Geometry check sheet. Reference: the model listing, model coordinates, mm. Face numbers are marked on the shaded views. Round coordinates to 2 decimals unless told otherwise and drop trailing zeros. Order: outer loops, then holes, each group sorted by start corner. A loop starts at its lowest first (then second) coordinate and runs counter-clockwise, first axis right, second up. Notation, with made-up numbers: (43, -0.5) - (75, -0.5) arc R28 ccw to (75, 21.5) - close; hole circle Ø9 at (33.25, -26). An arc over 180 degrees is marked (long way). Return JSON: item names as keys, results as strings. Group by question number.
Q1. Material ranges on line 1 along Y through (x, z) = (-5.5, 0.6); line 2 along Y through (x, z) = (-5, 1); line 3 along Z through (x, y) = (199, 3), recorded low to high.
Q2. Sectioned sample at B-B, the plane x = 130. Record the cut outline in (y, z).
Q3. Draft check along Y on the marked faces 1, 2 and 3. Enter one of: pulls with the +Y half, pulls with the -Y half, needs draft (parallel to the pull), parting line crosses it, or undercut.
Q4. Sectioned sample at A-A, the plane x = 307.5. Record the cut outline in (y, z).
Q5. Gauge pin test, flat ends, axial feed: pin 1 Ø3.5 at (x, z) = (340, 9) entering from -Y; pin 2 Ø2 at (x, z) = (-16, 7.5) entering from -Y; pin 3 Ø5 at (x, y) = (343, -4.5) entering from -Z; pin 4 Ø2.5 at (x, z) = (274, -24) entering from +Y. Record the tip position at first contact, or that the pin passes through.
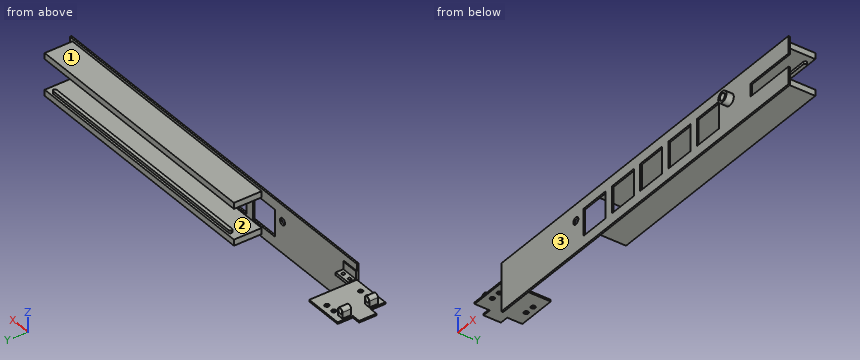
```python
from build123d import *

# Parameters (mm, degrees)
CROQUIS1_W               = 45
CROQUIS1_H               = 55
CROQUIS1_R               = 2.5
SALIENTE_EXTRUIR1_DEPTH  = 2
CROQUIS2_W               = 10
CROQUIS2_H               = 20
SALIENTE_EXTRUIR2_DEPTH  = 2
CROQUIS4_R               = 3
SALIENTE_EXTRUIR4_DEPTH  = 10
CROQUIS6_W               = 2
CROQUIS6_H               = 10
SALIENTE_EXTRUIR6_DEPTH  = 20
CROQUIS7_W               = 455
CROQUIS7_H               = 55
SALIENTE_EXTRUIR7_DEPTH  = 2
CROQUIS8_W               = 60
CROQUIS8_H               = 15
CORTAR_EXTRUIR1_DEPTH    = 2
SALIENTE_EXTRUIR8_DEPTH  = 20
CROQUIS10_R              = 1.75
CORTAR_EXTRUIR2_DEPTH    = 480.688961724
CROQUIS11_W              = 300
CROQUIS11_H              = 7
SALIENTE_EXTRUIR9_DEPTH  = 32
SALIENTE_EXTRUIR10_DEPTH = 3
CROQUIS17_R              = 4
CORTAR_EXTRUIR4_DEPTH    = 10
CROQUIS18_W              = 35
CROQUIS18_H              = 31
CORTAR_EXTRUIR5_DEPTH    = 10
CROQUIS19_R              = 4
CORTAR_EXTRUIR6_DEPTH    = 10
CROQUIS22_R              = 6.5
CROQUIS22_R_2            = 4
SALIENTE_EXTRUIR11_DEPTH = 8.5


with BuildPart() as part:
    # Croquis1 → Saliente-Extruir1 (new body)
    with BuildSketch(Plane.XY):
        Rectangle(CROQUIS1_W, CROQUIS1_H)
        with Locations((5.5, 19.5)):
            Circle(CROQUIS1_R, mode=Mode.SUBTRACT)
        with Locations((-5.5, 19.5)):
            Circle(CROQUIS1_R, mode=Mode.SUBTRACT)
        with Locations((-5.5, -19.5)):
            Circle(CROQUIS1_R, mode=Mode.SUBTRACT)
        with Locations((5.5, -19.5)):
            Circle(CROQUIS1_R, mode=Mode.SUBTRACT)
    extrude(amount=SALIENTE_EXTRUIR1_DEPTH)

    # Croquis2 → Saliente-Extruir2 (add)
    with BuildSketch(Plane(origin=(0, 0, 0), x_dir=(-1, 0, 0), z_dir=(0, 0, -1))):
        with Locations((27.5, 0)):
            Rectangle(CROQUIS2_W, CROQUIS2_H)
    extrude(amount=-SALIENTE_EXTRUIR2_DEPTH)

    # Croquis4 → Saliente-Extruir4 (add)
    with BuildSketch(Plane(origin=(0, -20.5, 0), x_dir=(-1, 0, 0), z_dir=(0, -1, 0))):
        with BuildLine():
            Line((13.5, -2), (20.5, -2))
            Line((20.5, -2), (20.5, -9))
            ThreePointArc((20.5, -9), (17, -12.5), (13.5, -9))
            Line((13.5, -9), (13.5, -2))
        make_face()
        with Locations(Location((17, -9, 0), (0, 0, 90))):
            Circle(CROQUIS4_R, mode=Mode.SUBTRACT)
    saliente_extruir4 = extrude(amount=-SALIENTE_EXTRUIR4_DEPTH)

    # Simetría1: Saliente-Extruir4 across plane
    add(saliente_extruir4.mirror(Plane.ZX))

    # Croquis6 → Saliente-Extruir6 (add)
    with BuildSketch(Plane(origin=(22.5, 0, 0), x_dir=(0, 0, -1), z_dir=(1, 0, 0))):
        with Locations((-1, -22.5)):
            Rectangle(CROQUIS6_W, CROQUIS6_H)
    extrude(amount=SALIENTE_EXTRUIR6_DEPTH)

    # Croquis7 → Saliente-Extruir7 (add)
    with BuildSketch(Plane(origin=(0, -27.5, 0), x_dir=(1, 0, 0), z_dir=(0, 1, 0))):
        with Locations((250, 7.5)):
            Rectangle(CROQUIS7_W, CROQUIS7_H)
    extrude(amount=-SALIENTE_EXTRUIR7_DEPTH)

    # Croquis8 → Cortar-Extruir1 (cut)
    with BuildSketch(Plane(origin=(0, -29.5, 0), x_dir=(-1, 0, 0), z_dir=(0, -1, 0))):
        with Locations((-447.5, 7.5)):
            Rectangle(CROQUIS8_W, CROQUIS8_H)
    extrude(amount=-CORTAR_EXTRUIR1_DEPTH, mode=Mode.SUBTRACT)

    # Croquis9 → Saliente-Extruir8 (add)
    with BuildSketch(Plane(origin=(42.5, 0, 0), x_dir=(0, 0, -1), z_dir=(1, 0, 0))):
        Polygon((-2, -26.357753354), (-2, -17.5), (-3.142246646, -17.5), (-3.142246646, -26.357753354), (-12, -26.357753354), (-12, -27.5), (-2, -27.5), align=None)
    extrude(amount=-SALIENTE_EXTRUIR8_DEPTH)

    # Croquis10 → Cortar-Extruir2 (cut, through all)
    with BuildSketch(Plane(origin=(0, 0, 0), x_dir=(-1, 0, 0), z_dir=(0, 0, -1))):
        with Locations((-26.5, -22)):
            Circle(CROQUIS10_R)
        with Locations((-36.5, -22)):
            Circle(CROQUIS10_R)
    extrude(amount=-CORTAR_EXTRUIR2_DEPTH, mode=Mode.SUBTRACT)

    # Croquis11 → Saliente-Extruir9 (add)
    with BuildSketch(Plane(origin=(0, -27.5, 0), x_dir=(1, 0, 0), z_dir=(0, 1, 0))):
        with Locations((323.5, 28.5)):
            Rectangle(CROQUIS11_W, CROQUIS11_H)
        with Locations((323.5, -13.5)):
            Rectangle(CROQUIS11_W, CROQUIS11_H)
    extrude(amount=SALIENTE_EXTRUIR9_DEPTH)

    # Croquis13 → Saliente-Extruir10 (add)
    with BuildSketch(Plane(origin=(0, 0, 10), x_dir=(-1, 0, 0), z_dir=(0, 0, -1))):
        with BuildLine():
            Line((-463.5, 2), (-185, 2))
            ThreePointArc((-185, 2), (-183.939339828, 1.560660172), (-183.5, 0.5))
            Line((-183.5, 0.5), (-183.5, -0.5))
            ThreePointArc((-183.5, -0.5), (-183.939339828, -1.560660172), (-185, -2))
            Line((-185, -2), (-463.5, -2))
            ThreePointArc((-463.5, -2), (-465.5, 0), (-463.5, 2))
        make_face()
    saliente_extruir10 = extrude(amount=SALIENTE_EXTRUIR10_DEPTH)

    # Simetría2: Saliente-Extruir10 across plane
    add(saliente_extruir10.mirror(Plane(origin=(0, 0, -7.5), x_dir=(1, 0, 0), z_dir=(0, 0, -1))))

    # Croquis17 → Cortar-Extruir4 (cut)
    with BuildSketch(Plane(origin=(0, -27.5, 0), x_dir=(1, 0, 0), z_dir=(0, 1, 0))):
        with Locations(Location((140.5, -1, 0), (0, 0, 270))):
            Circle(CROQUIS17_R)
    extrude(amount=-CORTAR_EXTRUIR4_DEPTH, mode=Mode.SUBTRACT)

    # Croquis18 → Cortar-Extruir5 (cut)
    with BuildSketch(Plane(origin=(0, -27.5, 0), x_dir=(1, 0, 0), z_dir=(0, 1, 0))):
        with Locations((170, 7.5)):
            Rectangle(CROQUIS18_W, CROQUIS18_H)
        with Locations((215, 7.5)):
            Rectangle(CROQUIS18_W, CROQUIS18_H)
        with Locations((260, 7.5)):
            Rectangle(CROQUIS18_W, CROQUIS18_H)
        with Locations((305, 7.5)):
            Rectangle(CROQUIS18_W, CROQUIS18_H)
        with Locations((350, 7.5)):
            Rectangle(CROQUIS18_W, CROQUIS18_H)
    extrude(amount=-CORTAR_EXTRUIR5_DEPTH, mode=Mode.SUBTRACT)

    # Croquis19 → Cortar-Extruir6 (cut)
    with BuildSketch(Plane(origin=(0, -27.5, 0), x_dir=(1, 0, 0), z_dir=(0, 1, 0))):
        with Locations(Location((384.5, 0, 0), (0, 0, 270))):
            Circle(CROQUIS19_R)
    extrude(amount=-CORTAR_EXTRUIR6_DEPTH, mode=Mode.SUBTRACT)

    # Croquis22 → Saliente-Extruir11 (add)
    with BuildSketch(Plane.XZ.offset(29.5)):
        with Locations(Location((384.5, 0, 0), (0, 0, 90))):
            Circle(CROQUIS22_R)
        with Locations(Location((384.5, 0, 0), (0, 0, 90))):
            Circle(CROQUIS22_R_2, mode=Mode.SUBTRACT)
    extrude(amount=SALIENTE_EXTRUIR11_DEPTH)


solid = part.part
```
Reply:
{
 "1": {"line 1": "-27.5 to -22, -17 to 17, 22 to 27.5", "line 2": "-27.5 to -21.95, -17.05 to 17.05, 21.95 to 27.5", "line 3": "-32 to -25, 10 to 17"},
 "2": {"outline": "(-29.5, -35) - (-27.5, -35) - (-27.5, 20) - (-29.5, 20) - close"},
 "3": {"face 1": "needs draft", "face 2": "undercut", "face 3": "pulls with the -Y half"},
 "4": {"outline": "(-29.5, -35) - (-27.5, -35) - (-27.5, -32) - (4.5, -32) - (4.5, -25) - (2, -25) - (2, -22) - (-2, -22) - (-2, -25) - (-27.5, -25) - (-27.5, -23) - (-29.5, -23) - close; (-29.5, 8) - (-27.5, 8) - (-27.5, 10) - (-2, 10) - (-2, 7) - (2, 7) - (2, 10) - (4.5, 10) - (4.5, 17) - (-27.5, 17) - (-27.5, 20) - (-29.5, 20) - close"},
 "5": {"pin 1": "y = -29.5", "pin 2": "through", "pin 3": "z = -32", "pin 4": "y = 4.5"}
}
